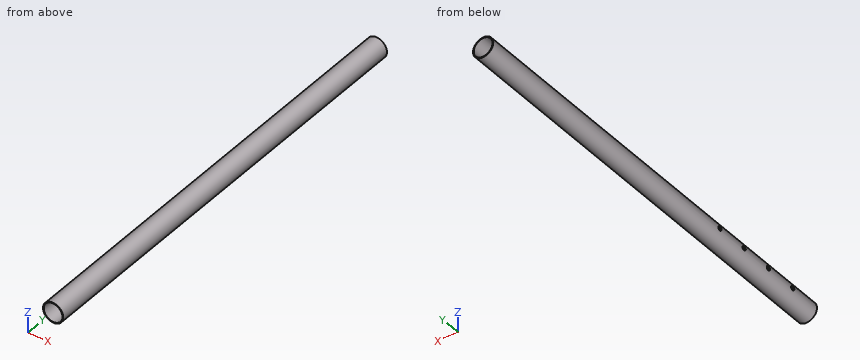
from build123d import *

# Parameters (mm, degrees)
SKETCH_1_R          = 19
SKETCH_1_R_2        = 17.5
EXTRUDE_1_DEPTH     = 800
SKETCH_2_R          = 4
CUT_EXTRUDE_1_DEPTH = 50


with BuildPart() as part:
    # 草图1 → 凸台-拉伸1 (new body)
    with BuildSketch(Plane(origin=(0, 0, 0), x_dir=(1, 0, 0), z_dir=(0, 1, 0))):
        with Locations(Location((0, 0, 0), (0, 0, 270))):
            Circle(SKETCH_1_R)
        with Locations(Location((0, 0, 0), (0, 0, 270))):
            Circle(SKETCH_1_R_2, mode=Mode.SUBTRACT)
    extrude(amount=EXTRUDE_1_DEPTH)

    # 草图2 → 切除-拉伸1 (cut)
    with BuildSketch(Plane(origin=(0, 0, 0), x_dir=(0, 0, -1), z_dir=(1, 0, 0))):
        with Locations((0, 60)):
            Circle(SKETCH_2_R)
        with Locations((0, 120)):
            Circle(SKETCH_2_R)
        with Locations((0, 180)):
            Circle(SKETCH_2_R)
        with Locations((0, 240)):
            Circle(SKETCH_2_R)
    extrude(amount=-CUT_EXTRUDE_1_DEPTH, mode=Mode.SUBTRACT)


solid = part.part
Here's how the part is built. I have some questions about the finished solid (model axes, mm). Give positions to 0.01 mm unless a question says otherwise; leave off trailing zeros. Loops run counter-clockwise (first coordinate to the right, second up) from the corner with the lowest first, then second, coordinate; pieces in that order, holes last. Notation, with made-up numbers: (30, 13) -> (44, 13) arc R18 ccw to (44, 25) -> close; hole circle Ø9 at (31, 43.5). An arc over 180 degrees is marked (long way). Answer as a JSON object with one key per item and string values. Group by question number.
Item 1: Imagine slicing it at A-A on x = 0. Write out the boundary of the cut face in (y, z), then the cut area to 3 significant figures.
Item 2: I need wall thicknesses on L1, parallel to Y at x = -17.95, z = 0; L2, parallel to X at y = 278.5, z = 0; L3, parallel to X at y = 203.5, z = -1.5. Which ranges of each line are inside material? Lowest first, please.
Item 3: Imagine slicing it at B-B on y = 145.5. Write out the boundary of the cut face in (x, z).
Item 4: Will these pins go through, and if not, where does the flat tip stop? pin 1 (7 mm diameter, centred on y = 60, z = 0, fed in from -X); pin 2 (12 mm diameter, centred on y = 607, z = 0.5, fed in from +X); pin 3 (6.5 mm diameter, centred on y = 180, z = 0, fed in from -X); pin 4 (21 mm diameter, centred on x = 0, z = 0, fed in from +Y).
Answer list:
{
 "1": {"outline": "(0, -19) -> (800, -19) -> (800, -17.5) -> (0, -17.5) -> close; (0, 17.5) -> (800, 17.5) -> (800, 19) -> (0, 19) -> close", "area": "2,400 mm2"},
 "2": {"L1": "y = 0 to 56, 64 to 116, 124 to 176, 184 to 236, 244 to 800", "L2": "x = -19 to -17.5, 17.5 to 19", "L3": "x = -18.94 to -17.44, 17.44 to 18.94"},
 "3": {"outline": "circle Ø38 at (0, 0); hole circle Ø35 at (0, 0)"},
 "4": {"pin 1": "stops at x = 17.15", "pin 2": "stops at x = 19", "pin 3": "stops at x = 17.2", "pin 4": "passes through"}
}
